For this review, use the dimensioned drawing (mm, ordinates from the lowest corner) and the shaded views. A direction names the side the tool comes from. Coordinates: 2 decimals unless noted, no trailing zeros. Order: outer loops, then holes, each group sorted by start corner. A loop starts at its lowest first (then second) coordinate and runs counter-clockwise, first axis right, second up. Notation, with made-up numbers: M 15,77 L 61,77 A10 ccw 61,93 Z; hole C 12,-14 d10. An arc over 180 degrees is marked long. Answer in a Markdown table with one row per item.
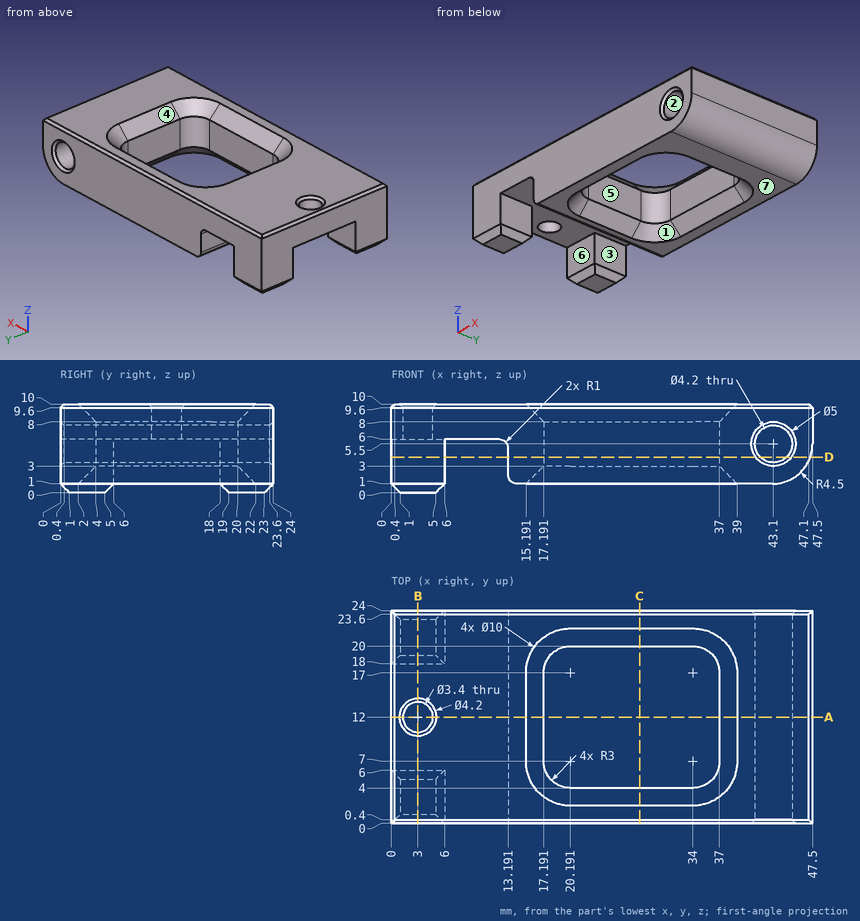
(1) Add section D-D, the plane z = 4. Give the number of separate pieces and of enclosed holes in the cut face, and give its area (3 significant figures).
Return value:
| item | result |
|---|---|
| separate pieces | 4 |
| enclosed holes | 1 |
| area | 509 mm2 |
(2) Add section B-B, the plane x = 3. Give the boundary of the cut face in (y, z), and give its area (3 significant figures).
Return value:
| item | result |
|---|---|
| outline | M 0,1 L 1,0 L 5,0 L 6,1 L 6,6 L 10.3,6 L 10.3,9.6 L 9.9,10 L 0.4,10 L 0,9.6 Z; M 13.7,6 L 18,6 L 18,1 L 19,0 L 23,0 L 24,1 L 24,9.6 L 23.6,10 L 14.1,10 L 13.7,9.6 Z |
| area | 152 mm2 |
(3) Draft analysis for pull direction Z (two halves, no side actions). For the marked faces 1, 2, 3 and 4, state which applies: pulls with the +Z half, pulls with the -Z half, needs draft (parallel to the pull), parting line crosses it, or undercut.
Return value:
| item | result |
|---|---|
| face 1 | pulls with the -Z half |
| face 2 | undercut |
| face 3 | needs draft |
| face 4 | pulls with the +Z half |
(4) For the marked faces 5, 6 and 7, list the 3-axis set-ups (+Z, -Z, +X, -X, +Y, -Y) from which the entire face can be reached by the end or side of a thin tool; tool diameter is ignored.
Return value:
| item | result |
|---|---|
| face 5 | +Z, -Z |
| face 6 | -Z, -X |
| face 7 | -Z, +X, +Y, -Y |
(5) For line 1 along Y through (x, z) = (3, 8.2); line 2 along Y through (x, z) = (27.5, 6.5); line 3 along X through (y, z) = (11.25, 6.5), list the stretches that pass through material, from the lowest coordinate up. Write a range as from..to.
Return value:
| item | result |
|---|---|
| line 1 | y = 0..10.3, 13.7..24 |
| line 2 | y = 0..4, 20..24 |
| line 3 | x = 0..1.47, 4.53..17.19, 37..41.25, 44.95..47.5 |
(6) Insertion check: pin 1 Ø3.5 at (y, z) = (14.5, 4) entering from -X; pin 2 Ø12 at (x, y) = (24.5, 8.5) entering from -Z; pin 3 Ø4.5 at (x, y) = (3, 12) entering from -Z. Each pin has a flat end and moves straight along its axis. Give the tip position at first contact, or say it passes through.
Return value:
| item | result |
|---|---|
| pin 1 | stops at x = 12.85 |
| pin 2 | stops at z = 1.5 |
| pin 3 | stops at z = 6 |
(7) Add section C-C, the plane x = 28. Give the boundary of the cut face in (y, z).
Return value:
| item | result |
|---|---|
| outline | M 0,1 L 2,1 L 4,3 L 4,8 L 2,10 L 0.4,10 L 0,9.6 Z; M 20,3 L 22,1 L 24,1 L 24,9.6 L 23.6,10 L 22,10 L 20,8 Z |
(8) Add section A-A, the plane y = 12. Give the boundary of the cut face in (x, z).
Return value:
| item | result |
|---|---|
| outline | M 0,6 L 1.3,6 L 1.3,9.6 L 0.9,10 L 0.4,10 L 0,9.6 Z; M 4.7,6 L 12.19,6 A1 cw 13.19,5 L 13.19,2 A1 ccw 14.19,1 L 15.19,1 L 17.19,3 L 17.19,8 L 15.19,10 L 5.1,10 L 4.7,9.6 Z; M 37,3 L 39,1 L 43,1 A4.5 ccw 47.5,5.5 L 47.5,9.6 L 47.1,10 L 39,10 L 37,8 Z; hole C 43.1,5.5 d4.2 |
